Job drawing, mm, ordinate dimensions from the low corner. One solid piece. A direction names the side the tool comes from. Round coordinates to 2 decimals unless told otherwise and drop trailing zeros. Loops run counter-clockwise (first coordinate to the right, second up) from the corner with the lowest first, then second, coordinate; pieces in that order, holes last. Notation, with made-up numbers: M -34,-18.5 L -24,-18.5 A14 ccw -24,6.5 Z; hole C 50.25,67 d10. An arc over 180 degrees is marked long. Use one line per item in the form item = value. Start each with the question number.
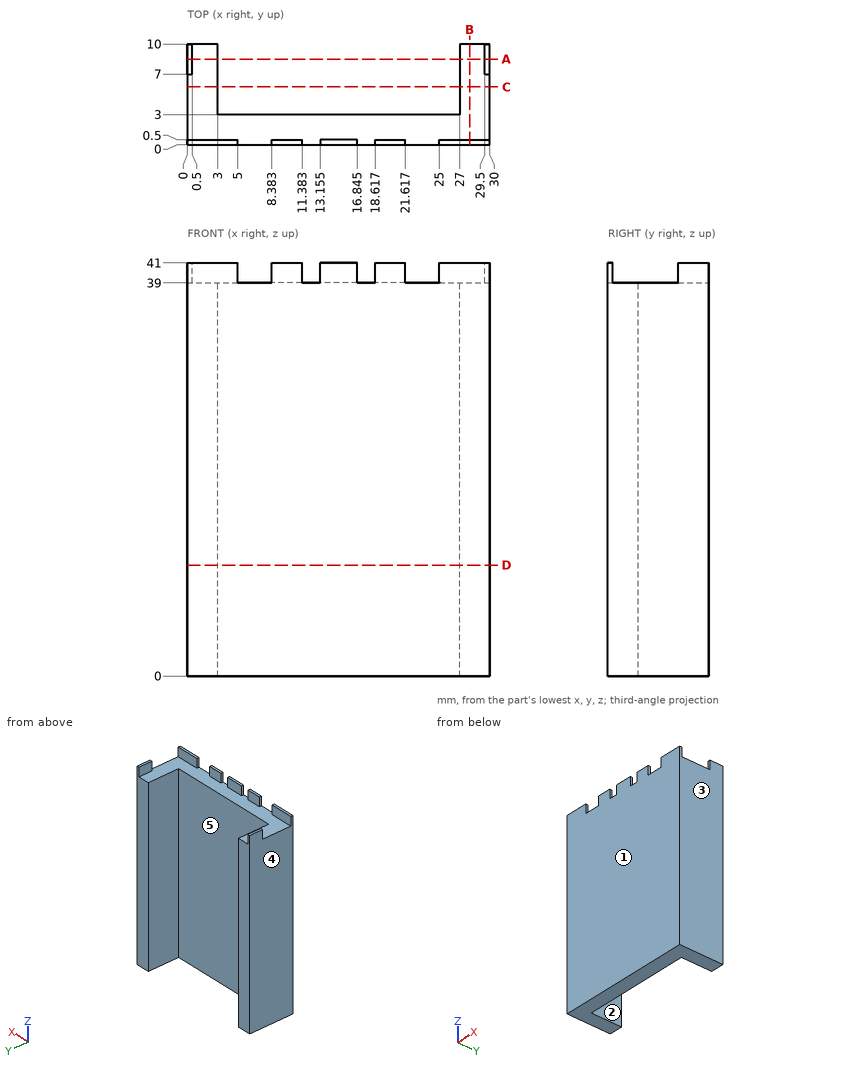
Q1. Tool access for the marked faces 1 and 2: list every direction of +Z, -Z, +X, -X, +Y, -Y with a clear straight run to the whole face (end or side of a thin tool).
Q2. Saw through at B-B (x = 28). Give the cut face in (y, z).
Q3. Drop flat-ended pins along their axis: P1, Ø5, axis at x = 10.5, z = 35.5, coming from the -Y side; P2, Ø2, axis at x = 14, z = 39.5, coming from the +Y side; P3, Ø0.6, axis at x = 9, z = 39.5, coming from the +Y side; P4, Ø3, axis at x = 26, y = 3.5, coming from the +Z side. Give the stop position or say it passes through.
Q4. Saw through at D-D (z = 11). Give the cut face in (x, y), and give its area (3 significant figures).
Q5. Pull direction X, two halves, no side cores. Call the marked faces 3, 4 and 5: pulls with the +X half, pulls with the -X half, needs draft (parallel to the pull), parting line crosses it, or undercut.
Q6. Wall check: probe 1 along X at (y, z) = (5.5, 6.5); probe 2 along Y at (x, z) = (4.5, 28.5); probe 3 along Z at (x, y) = (18.25, 0.5). Give the ranges that are in metal, low to high.
Q7. Saw through at C-C (y = 5.75). Give the cut face in (x, z), and give its area (3 significant figures).
Q8. Saw through at A-A (y = 8.5). Give the cut face in (x, z).
Filled in:
q1.face_1 = +Z, -Z, +X, -X, -Y
q1.face_2 = +Z, -Z, +Y
q2.outline = M 0,0 L 10,0 L 10,39 L 0.5,39 L 0.5,41 L 0,41 Z
q3.P1 = 0
q3.P2 = 3
q3.P3 = 0.5
q3.P4 = 39
q4.outline = M 0,0 L 30,0 L 30,10 L 27,10 L 27,3 L 3,3 L 3,10 L 0,10 Z
q4.area = 132 mm²
q5.face_3 = pulls with the +X half
q5.face_4 = pulls with the -X half
q5.face_5 = undercut
q6.probe_1 = 0 to 3, 27 to 30
q6.probe_2 = 0 to 3
q6.probe_3 = 0 to 39
q7.outline = M 0,0 L 3,0 L 3,39 L 0,39 Z; M 27,0 L 30,0 L 30,39 L 27,39 Z
q7.area = 234 mm²
q8.outline = M 0,0 L 3,0 L 3,39 L 0.5,39 L 0.5,41 L 0,41 Z; M 27,0 L 30,0 L 30,41 L 29.5,41 L 29.5,39 L 27,39 Z
